Part print with two shaded views. Sizes in mm from the minimum x, y, z corner. A direction names the side the tool comes from. Round coordinates to 2 decimals unless told otherwise and drop trailing zeros. Loops run counter-clockwise (first coordinate to the right, second up) from the corner with the lowest first, then second, coordinate; pieces in that order, holes last.
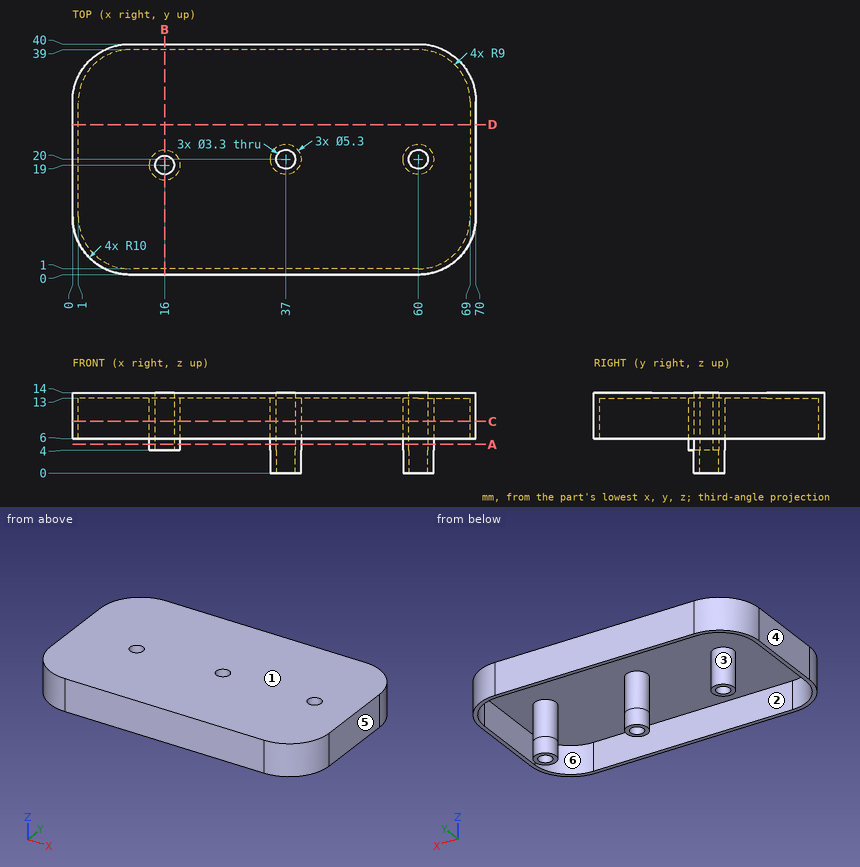
Item 1: 3-axis set-ups, long thin cutter, end or side, ignore diameter. For the marked faces 1 and 2: which of +Z, -Z, +X, -X, +Y, -Y reach the whole face in a straight line?
Verdict:
face 1: +Z, +X, -X, +Y, -Y
face 2: -Z
Item 2: Cut at D-D (y = 26). List the corners of the cut face in (x, z).
Verdict:
outline: (0, 6) - (1, 6) - (1, 13) - (69, 13) - (69, 6) - (70, 6) - (70, 14) - (0, 14) - close
Item 3: Cut at A-A (z = 5). List the corners of the cut face in (x, y).
Verdict:
outline: circle Ø5.3 at (16, 19); circle Ø5.3 at (37, 20); circle Ø5.3 at (60, 20); hole circle Ø3.3 at (16, 19); hole circle Ø3.3 at (37, 20); hole circle Ø3.3 at (60, 20)
Item 4: Wall check: L1, parallel to Y at x = 37, z = 6.5; L2, parallel to Y at x = 60, z = 2.45; L3, parallel to Y at x = 16, z = 9.5. Give the ranges that are in metal, low to high.
Verdict:
L1: y = 0 to 1, 17.35 to 18.35, 21.65 to 22.65, 39 to 40
L2: y = 17.35 to 18.35, 21.65 to 22.65
L3: y = 0 to 1, 16.35 to 17.35, 20.65 to 21.65, 39 to 40
Item 5: Cut at C-C (z = 9). List the corners of the cut face in (x, y), plus the area to 3 significant figures.
Verdict:
outline: (0, 10) arc R10 ccw to (10, 0) - (60, 0) arc R10 ccw to (70, 10) - (70, 30) arc R10 ccw to (60, 40) - (10, 40) arc R10 ccw to (0, 30) - close; circle Ø5.3 at (16, 19); circle Ø5.3 at (37, 20); circle Ø5.3 at (60, 20); hole (1, 10) arc R9 ccw to (10, 1) - (60, 1) arc R9 ccw to (69, 10) - (69, 30) arc R9 ccw to (60, 39) - (10, 39) arc R9 ccw to (1, 30) - close; hole circle Ø3.3 at (16, 19); hole circle Ø3.3 at (37, 20); hole circle Ø3.3 at (60, 20)
area: 240 mm2
Item 6: Flat gauge pins, fed straight in: P1, Ø2.5, axis at x = 60, y = 20, coming from the +Z side; P2, Ø4, axis at y = 7, z = 5.5, coming from the +X side; P3, Ø2.5, axis at x = 15.5, y = 19.5, coming from the -Z side. Where does each tip first touch, or does it go through?
Verdict:
P1: passes through
P2: stops at x = 69.94
P3: stops at z = 4
Item 7: Mould opens along X. For the marked faces 3, 4, 5 and 6 say: released by +X, released by -X, zero draft, split by the parting line, or undercut.
Verdict:
face 3: undercut
face 4: released by -X
face 5: released by +X
face 6: undercut
Item 8: Cut at B-B (x = 16). List the corners of the cut face in (y, z), plus the area to 3 significant figures.
Verdict:
outline: (0, 6) - (1, 6) - (1, 13) - (16.35, 13) - (16.35, 4) - (17.35, 4) - (17.35, 14) - (0, 14) - close; (20.65, 4) - (21.65, 4) - (21.65, 13) - (39, 13) - (39, 6) - (40, 6) - (40, 14) - (20.65, 14) - close
area: 68.7 mm2
